Design review of the part built by this model. Coordinates are the model's own, in mm. A direction names the side the tool comes from. Coordinates: 2 decimals unless noted, no trailing zeros. Loops run counter-clockwise (first coordinate to the right, second up) from the corner with the lowest first, then second, coordinate; pieces in that order, holes last. Notation, with made-up numbers: M -3.5,41.25 L 19.5,41.25 A22 ccw 19.5,62.25 Z; hole C -30,71.25 d2. An arc over 180 degrees is marked long. Put each result on its own line as item: value. Start each with the question number.
(1) The part is to be moulded in two halves that separate along Y. For faces 3 (the cylindrical face through (16.78, -20.8, -10.46)), 4 (the flat face through (33.1, 0, 0)), 5 (the flat face through (16, 22.615, 0)), 6 (the cylindrical face through (34.776, -9.006, 0.163)), say which applies: +Y half, -Y half, draft (parallel to the pull), parting line (faces both ways), or undercut.
(2) Take a section at B-B, the plane x = 2.5. Give the boundary of the cut face in (y, z) (3 decimals), then the cut area to 3 significant figures.
(3) Take a section at C-C, the plane y = 12.5. Give the boundary of the cut face in (x, z) (3 decimals), then the cut area to 3 significant figures.
(4) For faces 1 (the cylindrical face through (34.78, -7.27, 0.39)), 2 (the cylindrical face through (16.78, 20.71, 10.55)), list the 3-axis set-ups (+Z, -Z, +X, -X, +Y, -Y) from which the entire face can be reached by the end or side of a thin tool; tool diameter is ignored.
(5) Take a section at A-A, the plane z = 0. Give the boundary of the cut face in (x, y) (3 decimals).
(6) For probe 1 along Y at (x, z) = (35.4, 0) (3 decimals); probe 2 along X at (y, z) = (20, 10.25); probe 3 along Z at (x, y) = (12.5, -16.5), list the stretches that pass through material, from the lowest coordinate up. Write a range as [from, to].
(7) Clearance check with flat-ended pins moving along their axes: pin 1 (0.8 mm diameter, centred on y = -10, z = 0, fed in from +X); pin 2 (1.5 mm diameter, centred on y = -10.245, z = 0, fed in from -X). State where each tip first meets the part, or that it passes through.
(8) Take a section at D-D, the plane z = -9.25. Give the boundary of the cut face in (x, y), then the cut area to 3 significant figures.
```python
from build123d import *

# Parameters (mm, degrees)
SKETCH1_W           = 24.73
SKETCH1_H           = 45.23
BOSS_EXTRUDE1_DEPTH = 33.1
SKETCH2_R           = 3
SKETCH2_R_2         = 1.25
BOSS_EXTRUDE2_DEPTH = 3.4
FILLET1_R           = 6.35


with BuildPart() as part:
    # Sketch1 → Boss-Extrude1 (new body)
    with BuildSketch(Plane(origin=(0, 0, 0), x_dir=(0, 0, -1), z_dir=(1, 0, 0))):
        Rectangle(SKETCH1_W, SKETCH1_H)
    extrude(amount=BOSS_EXTRUDE1_DEPTH)

    # Sketch2 → Boss-Extrude2 (add)
    with BuildSketch(Plane(origin=(33.1, 0, 0), x_dir=(0, 0, -1), z_dir=(1, 0, 0))):
        with Locations((0, -10.245)):
            Circle(SKETCH2_R)
        with Locations((0, -10.245)):
            Circle(SKETCH2_R_2, mode=Mode.SUBTRACT)
    extrude(amount=BOSS_EXTRUDE2_DEPTH)

    # Fillet1
    fillet1_edges = [part.edges().sort_by_distance(p)[0] for p in [
        (16.55, -22.615, -12.365),
        (16.55, -22.615, 12.365),
        (16.55, 22.615, 12.365),
        (16.55, 22.615, -12.365),
    ]]
    fillet(fillet1_edges, radius=FILLET1_R)


solid = part.part
```
Computed values:
1. face 3: -Y half
1. face 4: draft
1. face 5: +Y half
1. face 6: undercut
2. outline: M -22.615,-6.015 A6.35 ccw -16.265,-12.365 L 16.265,-12.365 A6.35 ccw 22.615,-6.015 L 22.615,6.015 A6.35 ccw 16.265,12.365 L -16.265,12.365 A6.35 ccw -22.615,6.015 Z
2. area: 1,080 mm^2
3. outline: M 0,-12.365 L 33.1,-12.365 L 33.1,12.365 L 0,12.365 Z
3. area: 819 mm^2
4. face 1: +X
4. face 2: +Z, +X, -X, +Y
5. outline: M 0,-22.615 L 33.1,-22.615 L 33.1,-13.245 L 36.5,-13.245 L 36.5,-11.495 L 33.1,-11.495 L 33.1,-8.995 L 36.5,-8.995 L 36.5,-7.245 L 33.1,-7.245 L 33.1,22.615 L 0,22.615 Z
6. probe 1: y = [-13.245, -11.495], [-8.995, -7.245]
6. probe 2: x = [0, 33.1]
6. probe 3: z = [-12.36, 12.36]
7. pin 1: stops at x = 33.1
7. pin 2: stops at x = 0
8. outline: M 0,-21.73 L 33.1,-21.73 L 33.1,21.73 L 0,21.73 Z
8. area: 1,440 mm^2
